Input: part model. Units: mm. Frame: model coordinates. Face numbers are marked on the shaded views. A direction names the side the tool comes from. Give positions to 0.01 mm unless a question says otherwise; leave off trailing zeros. Loops run counter-clockwise (first coordinate to the right, second up) from the corner with the lowest first, then second, coordinate; pieces in that order, holes last. Notation, with made-up numbers: (-27.75, -1) -> (0.25, -1) arc R18 cw to (0.25, 21) -> close; hole circle Ø6 at (59.25, -14). An arc over 180 degrees is marked (long way). Answer as a JSON object with one key per item and string values.
```python
from build123d import *

# Parameters (mm, degrees)
SKETCH1_W           = 30
SKETCH1_H           = 30
BOSS_EXTRUDE1_DEPTH = 32.5
SKETCH2_W           = 15
SKETCH2_H           = 20
BOSS_EXTRUDE2_DEPTH = 10
CHAMFER1_SIZE       = 3


with BuildPart() as part:
    # Sketch1 → Boss-Extrude1 (new body, symmetric)
    with BuildSketch(Plane.XY):
        Polygon((-17.5, 27.5), (17.5, 27.5), (17.5, 17.5), (27.5, 17.5), (27.5, -17.5), (17.5, -17.5), (17.5, -27.5), (-17.5, -27.5), (-17.5, -17.5), (-27.5, -17.5), (-27.5, 17.5), (-17.5, 17.5), align=None)
        Rectangle(SKETCH1_W, SKETCH1_H, mode=Mode.SUBTRACT)
    extrude(amount=BOSS_EXTRUDE1_DEPTH, both=True)

    # Sketch2 → Boss-Extrude2 (add)
    with BuildSketch(Plane(origin=(27.5, 0, 0), x_dir=(0, 0, -1), z_dir=(1, 0, 0))):
        with Locations((25, -2.5)):
            Rectangle(SKETCH2_W, SKETCH2_H)
    extrude(amount=BOSS_EXTRUDE2_DEPTH)

    # Chamfer1
    chamfer1_edges = [part.edges().sort_by_distance(p)[0] for p in [
        (37.5, -2.5, -32.5),
        (37.5, 7.5, -25),
        (37.5, -12.5, -25),
    ]]
    chamfer(chamfer1_edges, length=CHAMFER1_SIZE)


solid = part.part
```
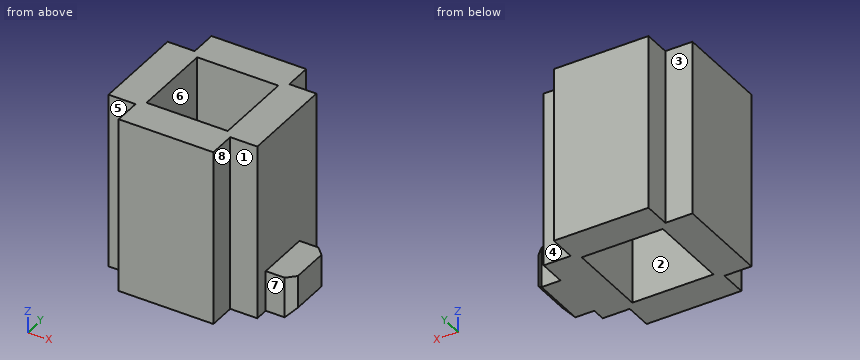
Q1. Access query for the marked faces 1, 2, 3, 4 and 5. Directions: +Z, -Z, +X, -X, +Y, -Y. A direction counts if a zero-diameter tool reaches every point of the face in a straight line with its end or side. Return the directions, or none.
Evaluation:
{"face 1": "+Z, -Z, +X, -Y", "face 2": "+Z, -Z", "face 3": "+Z, -Z, -X, +Y", "face 4": "+Z, -Z, +X, +Y", "face 5": "+Z, -Z, -X, -Y"}
Q2. Section C-C, the plane z = 23.5. Return the cut outline in (x, y), then the cut area to 4 significant figures.
Evaluation:
{"outline": "(-27.5, -17.5) -> (-17.5, -17.5) -> (-17.5, -27.5) -> (17.5, -27.5) -> (17.5, -17.5) -> (27.5, -17.5) -> (27.5, 17.5) -> (17.5, 17.5) -> (17.5, 27.5) -> (-17.5, 27.5) -> (-17.5, 17.5) -> (-27.5, 17.5) -> close; hole (-15, -15) -> (15, -15) -> (15, 15) -> (-15, 15) -> close", "area": "1,725 mm2"}
Q3. Ray query, line 1 along Y through (x, z) = (-1.5, 0.5); line 2 along Y through (x, z) = (20, 4.5). Return the intervals inside material, ascending.
Evaluation:
{"line 1": "y = -27.5 to -15, 15 to 27.5", "line 2": "y = -17.5 to 17.5"}
Q4. Section B-B, the plane x = 1. Return the cut outline in (y, z), then the cut area to 4 significant figures.
Evaluation:
{"outline": "(-27.5, -32.5) -> (-15, -32.5) -> (-15, 32.5) -> (-27.5, 32.5) -> close; (15, -32.5) -> (27.5, -32.5) -> (27.5, 32.5) -> (15, 32.5) -> close", "area": "1,625 mm2"}
Q5. Pin query (flat end, axial travel): pin 1 (2 mm diameter, centred on x = 31, z = -27.5, fed in from +Y); pin 2 (5 mm diameter, centred on x = 21.5, z = 11, fed in from -Y); pin 3 (5 mm diameter, centred on y = 21, z = -7.5, fed in from +X). Return the tip coordinate at first contact, or that it passes through.
Evaluation:
{"pin 1": "stops at y = 7.5", "pin 2": "stops at y = -17.5", "pin 3": "stops at x = 17.5"}
Q6. Section D-D, the plane z = -23.5. Return the cut outline in (x, y), then the cut area to 3 significant figures.
Evaluation:
{"outline": "(-27.5, -17.5) -> (-17.5, -17.5) -> (-17.5, -27.5) -> (17.5, -27.5) -> (17.5, -17.5) -> (27.5, -17.5) -> (27.5, -12.5) -> (34.5, -12.5) -> (37.5, -9.5) -> (37.5, 4.5) -> (34.5, 7.5) -> (27.5, 7.5) -> (27.5, 17.5) -> (17.5, 17.5) -> (17.5, 27.5) -> (-17.5, 27.5) -> (-17.5, 17.5) -> (-27.5, 17.5) -> close; hole (-15, -15) -> (15, -15) -> (15, 15) -> (-15, 15) -> close", "area": "1,920 mm2"}
Q7. Draft query along X for the marked faces 6, 7 and 8. Return one class per face: +X half, -X half, draft (parallel to the pull), parting line (faces both ways), or undercut.
Evaluation:
{"face 6": "undercut", "face 7": "draft", "face 8": "+X half"}
Q8. Section A-A, the plane y = -2.5. Return the cut outline in (x, z), then the cut area to 3 significant figures.
Evaluation:
{"outline": "(-27.5, -32.5) -> (-15, -32.5) -> (-15, 32.5) -> (-27.5, 32.5) -> close; (15, -32.5) -> (34.5, -32.5) -> (37.5, -29.5) -> (37.5, -17.5) -> (27.5, -17.5) -> (27.5, 32.5) -> (15, 32.5) -> close", "area": "1,770 mm2"}
